Geometry check sheet. Reference: the model listing, model coordinates, mm. A direction names the side the tool comes from. Give positions to 0.01 mm unless a question says otherwise; leave off trailing zeros. Loops run counter-clockwise (first coordinate to the right, second up) from the corner with the lowest first, then second, coordinate; pieces in that order, holes last.
1. Material ranges on L1, parallel to Z at x = -10.5, y = 25.6; L2, parallel to Y at x = 21.8, z = 72.9; L3, parallel to Z at x = -8, y = -28.65, recorded low to high.
2. Cross-section at B-B, the plane x = -18. Record the cut outline in (y, z).
3. Cross-section at A-A, the plane y = 18. Record the cut outline in (x, z).
4. Go/stop test with flat-tipped pins: pin 1 Ø8 at (x, y) = (12.5, 21) entering from +Z; pin 2 Ø1.6 at (y, z) = (4.94, 72.9) entering from +X. Record where each tip stops, or that it passes through.
5. Release check for a two-part mould opening along Z. For faces 4 (the cylindrical face through (-22.972, -10.724, 2.57)), 5 (the flat face through (-25, -1, 42)) record: +Z half, -Z half, draft (parallel to the pull), parting line (faces both ways), or undercut.
6. Tool access check on faces 1 (the cylindrical face through (23, 9.9, 73.9)), 2 (the cylindrical face through (0.44, -25.94, 71.25)), 3 (the cylindrical face through (10.5, 25.5, 78.9)). Record the directions out of +Z, -Z, +X, -X, +Y, -Y that give a thin tool (end or side, any length) a straight path to the whole face; none if there is none.
from build123d import *

# Parameters (mm, degrees)
BOSS_EXTRUDE1_DEPTH                    = 85.399999968
SKETCH2_R                              = 19.3
SKETCH2_R_2                            = 17.008
BOSS_EXTRUDE2_DEPTH                    = 2.5
DRAFT1_ANGLE                           = 15
DOME1_FACE_RADIUS                      = 16.338127019
DOME1_HEIGHT                           = 1
F_2_0_2_DIAMETER_HOLE1_D               = 2
F_2_0_2_DIAMETER_HOLE1_DEPTH           = 4
F_2_0_2_DIAMETER_HOLE1_TIP             = 0.600860619
F_2_0_2_DIAMETER_HOLE1_ON_FACE_2_D     = 2
F_2_0_2_DIAMETER_HOLE1_ON_FACE_2_DEPTH = 4
F_2_0_2_DIAMETER_HOLE1_ON_FACE_2_TIP   = 0.600860619
F_2_0_2_DIAMETER_HOLE1_ON_FACE_3_D     = 2
F_2_0_2_DIAMETER_HOLE1_ON_FACE_3_DEPTH = 4
F_2_0_2_DIAMETER_HOLE1_ON_FACE_3_TIP   = 0.600860619
F_2_0_2_DIAMETER_HOLE1_ON_FACE_4_D     = 2
F_2_0_2_DIAMETER_HOLE1_ON_FACE_4_DEPTH = 4
F_2_0_2_DIAMETER_HOLE1_ON_FACE_4_TIP   = 0.600860619
F_1_4_CLEARANCE_HOLE1_D                = 6.7564
F_1_4_CLEARANCE_HOLE1_DEPTH            = 8
F_1_4_CLEARANCE_HOLE1_TIP              = 2.029827343


with BuildPart() as part:
    # Sketch1 → Boss-Extrude1 (new body)
    with BuildSketch(Plane.XY):
        Polygon((-25, 25.5), (-23, 27.5), (23, 27.5), (25, 25.5), (25, -28), (23, -30), (-21, -30), (-25, -26), align=None)
    extrude(amount=BOSS_EXTRUDE1_DEPTH)

    # Sketch2 → Boss-Extrude2 (add)
    with BuildSketch(Plane.XY.offset(85.399999968)):
        with Locations(Location((0, 0, 0), (0, 0, 180))):
            Circle(SKETCH2_R)
        Circle(SKETCH2_R_2, mode=Mode.SUBTRACT)
    extrude(amount=BOSS_EXTRUDE2_DEPTH)

    # Draft1
    draft1_faces = [part.faces().sort_by_distance(p)[0] for p in [
        (-17.008, 0, 86.649999968),
    ]]
    draft(draft1_faces, Plane.XY.offset(87.899999968), DRAFT1_ANGLE)

    # Dome1: a dome of height H over a round flat face of radius A is a cap of a sphere of radius (A * A + H * H) / (2 * H)
    dome1_r = (DOME1_FACE_RADIUS * DOME1_FACE_RADIUS + DOME1_HEIGHT * DOME1_HEIGHT) / (2 * DOME1_HEIGHT)
    dome1_base = Plane((0, 0, 85.399999968), z_dir=(0, 0, 1))
    with Locations(dome1_base.offset(DOME1_HEIGHT - dome1_r)):
        dome1_ball = Sphere(dome1_r, mode=Mode.PRIVATE)
    add(split(dome1_ball, bisect_by=dome1_base, keep=Keep.TOP, mode=Mode.PRIVATE))

    # Ø2.0 (2) Diameter Hole1
    with Locations(Plane(origin=(25, 9.899748742, 72.899999968), x_dir=(0, 0, 1), z_dir=(1, 0, 0))):
        with Locations((0, 0), (-20, 0), (0, 4.956938323), (0, 20), (-20, 4.956938323), (-20, 20), (-20, 24.956938323), (-48, 0), (-48, 20)):
            Hole(F_2_0_2_DIAMETER_HOLE1_D / 2, depth=F_2_0_2_DIAMETER_HOLE1_DEPTH)
            with Locations((0, 0, -(F_2_0_2_DIAMETER_HOLE1_DEPTH + F_2_0_2_DIAMETER_HOLE1_TIP / 2))):  # 118° drill point
                Cone(0, F_2_0_2_DIAMETER_HOLE1_D / 2, F_2_0_2_DIAMETER_HOLE1_TIP, mode=Mode.SUBTRACT)

    # Ø2.0 (2) Diameter Hole1 on face 2
    with Locations(Plane(origin=(-25, -9.732668619, 2.699999968), x_dir=(0, 0, -1), z_dir=(-1, 0, 0))):
        with Locations((0, 0), (0, -14)):
            Hole(F_2_0_2_DIAMETER_HOLE1_ON_FACE_2_D / 2, depth=F_2_0_2_DIAMETER_HOLE1_ON_FACE_2_DEPTH)
            with Locations((0, 0, -(F_2_0_2_DIAMETER_HOLE1_ON_FACE_2_DEPTH + F_2_0_2_DIAMETER_HOLE1_ON_FACE_2_TIP / 2))):  # 118° drill point
                Cone(0, F_2_0_2_DIAMETER_HOLE1_ON_FACE_2_D / 2, F_2_0_2_DIAMETER_HOLE1_ON_FACE_2_TIP, mode=Mode.SUBTRACT)

    # Ø2.0 (2) Diameter Hole1 on face 3
    with Locations(Plane(origin=(-10.5, 27.5, 77.899999968), x_dir=(0, 0, 1), z_dir=(0, 1, 0))):
        with Locations((0, 0), (0, 21), (-48.3, 25.4), (-73, 0)):
            Hole(F_2_0_2_DIAMETER_HOLE1_ON_FACE_3_D / 2, depth=F_2_0_2_DIAMETER_HOLE1_ON_FACE_3_DEPTH)
            with Locations((0, 0, -(F_2_0_2_DIAMETER_HOLE1_ON_FACE_3_DEPTH + F_2_0_2_DIAMETER_HOLE1_ON_FACE_3_TIP / 2))):  # 118° drill point
                Cone(0, F_2_0_2_DIAMETER_HOLE1_ON_FACE_3_D / 2, F_2_0_2_DIAMETER_HOLE1_ON_FACE_3_TIP, mode=Mode.SUBTRACT)

    # Ø2.0 (2) Diameter Hole1 on face 4
    with Locations(Plane(origin=(8, -30, 22.899999968), x_dir=(0, 0, -1), z_dir=(0, -1, 0))):
        with Locations((0, 0), (0, -16), (-29, -16), (-29, 0), (-24.8, 5.5), (-24.8, -21.5), (8.2, 5.5), (8.2, -21.5)):
            Hole(F_2_0_2_DIAMETER_HOLE1_ON_FACE_4_D / 2, depth=F_2_0_2_DIAMETER_HOLE1_ON_FACE_4_DEPTH)
            with Locations((0, 0, -(F_2_0_2_DIAMETER_HOLE1_ON_FACE_4_DEPTH + F_2_0_2_DIAMETER_HOLE1_ON_FACE_4_TIP / 2))):  # 118° drill point
                Cone(0, F_2_0_2_DIAMETER_HOLE1_ON_FACE_4_D / 2, F_2_0_2_DIAMETER_HOLE1_ON_FACE_4_TIP, mode=Mode.SUBTRACT)

    # 1/4 Clearance Hole1
    with Locations(Plane.XZ.offset(30)):
        with Locations((0, 67.899999968)):
            Hole(F_1_4_CLEARANCE_HOLE1_D / 2, depth=F_1_4_CLEARANCE_HOLE1_DEPTH)
            with Locations((0, 0, -(F_1_4_CLEARANCE_HOLE1_DEPTH + F_1_4_CLEARANCE_HOLE1_TIP / 2))):  # 118° drill point
                Cone(0, F_1_4_CLEARANCE_HOLE1_D / 2, F_1_4_CLEARANCE_HOLE1_TIP, mode=Mode.SUBTRACT)


solid = part.part
Result:
1. L1: z = 0 to 3.9, 5.9 to 76.9, 78.9 to 85.4
1. L2: y = -30 to -11.1, -9.1 to 3.94, 5.94 to 8.9, 10.9 to 27.5
1. L3: z = 0 to 21.9, 23.9 to 50.9, 52.9 to 85.4
2. outline: (-30, 0) - (27.5, 0) - (27.5, 85.4) - (6.96, 85.4) - (6.96, 87.9) - (-6.96, 87.9) - (-6.96, 85.4) - (-30, 85.4) - close
3. outline: (-25, 0) - (25, 0) - (25, 85.4) - (6.96, 85.4) - (6.96, 87.9) - (-6.96, 87.9) - (-6.96, 85.4) - (-25, 85.4) - close
4. pin 1: stops at z = 85.4
4. pin 2: stops at x = 20.88
5. face 4: undercut
5. face 5: draft
6. face 1: +X
6. face 2: -Y
6. face 3: +Y
